```python
from build123d import *

# Parameters (mm, degrees)
SKETCH1_R               = 35
BOSS_EXTRUDE1_DEPTH     = 5
BOSS_EXTRUDE2_DEPTH     = 35
SKETCH3_W               = 30
SKETCH3_H               = 5
BOSS_EXTRUDE3_DEPTH     = 25
SKETCH4_W               = 3
SKETCH4_H               = 30
BOSS_EXTRUDE5_DEPTH     = 5
CUT_EXTRUDE1_DEPTH      = 38
CUT_EXTRUDE1_DEPTH_BACK = 61.621778265
SKETCH5_R               = 1
FILLET1_R               = 1
FILLET2_R               = 1
FILLET3_R               = 1
CUT_EXTRUDE2_REACH      = 65.64
CUT_EXTRUDE2_END_RADIUS = 1
SKETCH6_R               = 0.5


with BuildPart() as part:
    # Sketch1 → Boss-Extrude1 (new body)
    with BuildSketch(Plane.XY):
        Circle(SKETCH1_R)
    extrude(amount=-BOSS_EXTRUDE1_DEPTH)

    # Sketch2 → Boss-Extrude2 (add)
    with BuildSketch(Plane.XY):
        with BuildLine():
            Line((-15, -15), (15, -15))
            ThreePointArc((15, -15), (14.863587797, -17.018355219), (14.456832295, -19))
            Line((14.456832295, -19), (-14.456832295, -19))
            ThreePointArc((-14.456832295, -19), (-14.863587797, -17.018355219), (-15, -15))
        make_face()
    extrude(amount=BOSS_EXTRUDE2_DEPTH)

    # Sketch3 → Boss-Extrude3 (add)
    with BuildSketch(Plane(origin=(0, -15, 0), x_dir=(1, 0, 0), z_dir=(0, 1, 0))):
        with Locations((0, -32.5)):
            Rectangle(SKETCH3_W, SKETCH3_H)
    extrude(amount=BOSS_EXTRUDE3_DEPTH)

    # Sketch4 → Boss-Extrude5 (add)
    with BuildSketch(Plane(origin=(0, -15, 0), x_dir=(1, 0, 0), z_dir=(0, 1, 0))):
        with Locations((9, -15)):
            Rectangle(SKETCH4_W, SKETCH4_H)
        with Locations((-9, -15)):
            Rectangle(SKETCH4_W, SKETCH4_H)
    extrude(amount=BOSS_EXTRUDE5_DEPTH)

    # Sketch5 → Cut-Extrude1 (cut, two sides: drawn at the far end of the back side and taken through both)
    with BuildSketch(Plane(origin=(0, 0, 0), x_dir=(1, 0, 0), z_dir=(0, 1, 0)).offset(-CUT_EXTRUDE1_DEPTH_BACK)):
        with Locations(Location((0, 2.5, 0), (0, 0, 90))):
            Circle(SKETCH5_R)
    extrude(amount=CUT_EXTRUDE1_DEPTH + CUT_EXTRUDE1_DEPTH_BACK, mode=Mode.SUBTRACT)

    # Fillet1
    fillet1_edges = [part.edges().sort_by_distance(p)[0] for p in [
        (15, 10, 32.5),
        (-15, 10, 32.5),
    ]]
    fillet(fillet1_edges, radius=FILLET1_R)

    # Fillet2
    fillet2_edges = [part.edges().sort_by_distance(p)[0] for p in [
        (7.5, -15, 15),
        (-7.5, -15, 15),
    ]]
    fillet(fillet2_edges, radius=FILLET2_R)

    # Fillet3
    fillet3_edges = [part.edges().sort_by_distance(p)[0] for p in [
        (10.5, -15, 15),
        (-10.5, -15, 15),
    ]]
    fillet(fillet3_edges, radius=FILLET3_R)

    # Cut-Extrude2: up to this cylinder (the profile starts outside it)
    cut_extrude2_end = Plane(origin=(0, 0, -2.5), z_dir=(0, -1, 0)) * Cylinder(CUT_EXTRUDE2_END_RADIUS, 156.28, mode=Mode.PRIVATE)
    # Sketch6 → Cut-Extrude2 (cut, up to the surface)
    with BuildSketch(Plane(origin=(0, 0, -5), x_dir=(-1, 0, 0), z_dir=(0, 0, -1)), mode=Mode.PRIVATE) as cut_extrude2_sk1:
        with Locations((0, 11)):
            Circle(SKETCH6_R)
    cut_extrude2_tool1 = extrude(cut_extrude2_sk1.sketch, amount=-CUT_EXTRUDE2_REACH, mode=Mode.PRIVATE) - cut_extrude2_end
    add(cut_extrude2_tool1.solids().sort_by_distance((0, 11, -5))[0], mode=Mode.SUBTRACT)
    # Sketch6 → Cut-Extrude2 (cut, up to the surface)
    with BuildSketch(Plane(origin=(0, 0, -5), x_dir=(-1, 0, 0), z_dir=(0, 0, -1)), mode=Mode.PRIVATE) as cut_extrude2_sk2:
        with Locations((0, -11)):
            Circle(SKETCH6_R)
    cut_extrude2_tool2 = extrude(cut_extrude2_sk2.sketch, amount=-CUT_EXTRUDE2_REACH, mode=Mode.PRIVATE) - cut_extrude2_end
    add(cut_extrude2_tool2.solids().sort_by_distance((0, -11, -5))[0], mode=Mode.SUBTRACT)


solid = part.part
```
Model file for the job. Use its own axes, mm. A direction names the side the tool comes from. Round coordinates to 2 decimals unless told otherwise and drop trailing zeros. Order: outer loops, then holes, each group sorted by start corner. A loop starts at its lowest first (then second) coordinate and runs counter-clockwise, first axis right, second up. Notation, with made-up numbers: M -17.75,23.5 L 32.25,23.5 A15 cw 32.25,48.5 Z; hole C 48,40 d9. An arc over 180 degrees is marked long. Use CSV: the item, a comma, the result in double quotes.
Item 1: Saw through at B-B (z = 18). List the corners of the cut face in (x, y).
Worked answers:
outline,"M -15,-15 A15 ccw -14.46,-19 L 14.46,-19 A15 ccw 15,-15 L 11.5,-15 A1 cw 10.5,-14 L 10.5,-10 L 7.5,-10 L 7.5,-14 A1 cw 6.5,-15 L -6.5,-15 A1 cw -7.5,-14 L -7.5,-10 L -10.5,-10 L -10.5,-14 A1 cw -11.5,-15 Z"
Item 2: Which spindle directions (+Z, -Z, +X, -X, +Y, -Y) get a long thin tool onto all of the face, cutting with end or side? Do faces 1 (the face through (0, -19, 17)), 2 (the face through (-10.5, -12, 15)), 3 (the face through (9, -10, 15)), 4 (the face through (7.5, -12, 15)). Say none if no direction does.
Worked answers:
face 1,"+Z, +X, -X, -Y"
face 2,"-X, +Y"
face 3,"+X, -X, +Y"
face 4,"+Y"
Item 3: Pull direction Z, two halves, no side cores. Call faces 5 (the face through (0, 0, -5)), 6 (the face through (-15, -3, 33)), 7 (the face through (-13, -15, 15)): released by +Z, released by -Z, zero draft, split by the parting line, or undercut.
Worked answers:
face 5,"released by -Z"
face 6,"zero draft"
face 7,"undercut"
Item 4: Probe probe 1 along Y at (x, z) = (0, -3.85); probe 2 along X at (y, z) = (-12.5, 12); probe 3 along Z at (x, y) = (13, 3). List the from-to ranges inside material, lowest first.
Worked answers:
probe 1,"-35 to -11.5, -10.5 to 10.5, 11.5 to 35"
probe 2,"-10.5 to -7.5, 7.5 to 10.5"
probe 3,"-5 to 0, 30 to 35"
Item 5: Pin check, flat tips, straight feed: pin 1 (6.5 mm diameter, centred on x = 2, z = 12.5, fed in from +Y); pin 2 (2.5 mm diameter, centred on x = 8.5, z = 20, fed in from +Y); pin 3 (1.5 mm diameter, centred on x = 4.5, z = 33, fed in from +Y). Stop position of each tip, or through.
Worked answers:
pin 1,"y = -15"
pin 2,"y = -10"
pin 3,"y = 10"
Item 6: Saw through at D-D (y = -16). List the corners of the cut face in (x, z).
Worked answers:
outline,"M -31.13,-5 L 31.13,-5 L 31.13,0 L 14.97,0 L 14.97,35 L -14.97,35 L -14.97,0 L -31.13,0 Z; hole C 0,-2.5 d2"
Item 7: Saw through at A-A (y = 21). List the corners of the cut face in (x, z), plus the area to 3 significant figures.
Worked answers:
outline,"M -28,-5 L 28,-5 L 28,0 L -28,0 Z; hole C 0,-2.5 d2"
area,"277 mm²"
Item 8: Saw through at C-C (x = 2.5). List the corners of the cut face in (y, z), plus the area to 3 significant figures.
Worked answers:
outline,"M -34.91,-5 L 34.91,-5 L 34.91,0 L -15,0 L -15,30 L 10,30 L 10,35 L -19,35 L -19,0 L -34.91,0 Z"
area,"614 mm²"
